The model under review builds one solid part; all positions refer to its coordinate system, in mm. Face numbers are marked on the shaded views. A direction names the side the tool comes from. Coordinates: 2 decimals unless noted, no trailing zeros. Order: outer loops, then holes, each group sorted by start corner. A loop starts at its lowest first (then second) coordinate and runs counter-clockwise, first axis right, second up. Notation, with made-up numbers: M 26,26 L 53,26 A12 cw 53,34 Z; hole C 73.25,21 d1. An arc over 180 degrees is marked long. One line per item, written item: value.
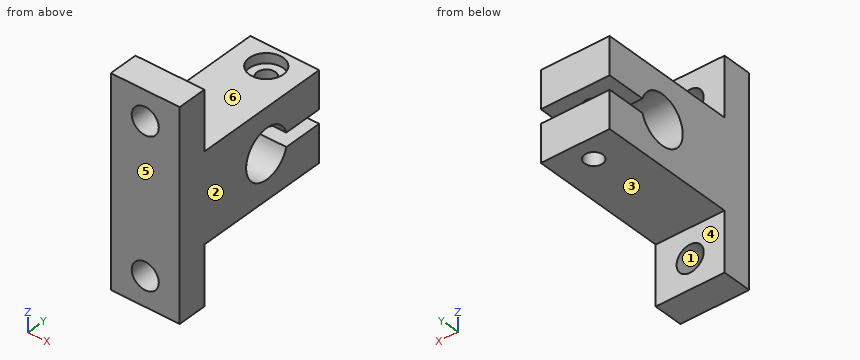
```python
from build123d import *

# Parameters (mm, degrees)
BOSS_EXTRUDE1_DEPTH = 14
SKETCH3_R           = 1.85
CUT_EXTRUDE1_DEPTH  = 48.455242071
SKETCH4_R           = 2.75
CUT_EXTRUDE2_DEPTH  = 53.383203415
SKETCH5_R           = 3.452522479
CUT_EXTRUDE3_DEPTH  = 2


with BuildPart() as part:
    # Sketch2 → Boss-Extrude1 (new body)
    with BuildSketch(Plane(origin=(0, 0, 0), x_dir=(0, 0, -1), z_dir=(1, 0, 0))):
        with BuildLine():
            Line((0, 0), (42, 0))
            Line((42, 0), (42, 6))
            Line((42, 6), (30, 6))
            Line((30, 6), (30, 34))
            Line((30, 34), (22.4, 34))
            Line((22.4, 34), (22.4, 26))
            ThreePointArc((22.4, 26), (21, 16.2), (19.6, 26))
            Line((19.6, 26), (19.6, 34))
            Line((19.6, 34), (12, 34))
            Line((12, 34), (12, 6))
            Line((12, 6), (0, 6))
            Line((0, 6), (0, 0))
        make_face()
    extrude(amount=BOSS_EXTRUDE1_DEPTH)

    # Sketch3 → Cut-Extrude1 (cut, through all)
    with BuildSketch(Plane(origin=(0, 0, -30), x_dir=(-1, 0, 0), z_dir=(0, 0, -1))):
        with Locations((-7, 29.5)):
            Circle(SKETCH3_R)
    extrude(amount=-CUT_EXTRUDE1_DEPTH, mode=Mode.SUBTRACT)

    # Sketch4 → Cut-Extrude2 (cut, through all)
    with BuildSketch(Plane(origin=(0, 6, 0), x_dir=(1, 0, 0), z_dir=(0, 1, 0))):
        with Locations(Location((7, 36, 0), (0, 0, 270))):
            Circle(SKETCH4_R)
        with Locations(Location((7, 6, 0), (0, 0, 270))):
            Circle(SKETCH4_R)
    extrude(amount=-CUT_EXTRUDE2_DEPTH, mode=Mode.SUBTRACT)

    # Sketch5 → Cut-Extrude3 (cut)
    with BuildSketch(Plane.XY.offset(-12)):
        with Locations((7, 29.5)):
            Circle(SKETCH5_R)
    extrude(amount=-CUT_EXTRUDE3_DEPTH, mode=Mode.SUBTRACT)


solid = part.part
```
(1) Tool access review of the marked faces 4, 5 and 6: name each direction out of +Z, -Z, +X, -X, +Y, -Y from which nothing blocks a thin tool from reaching the whole face with its end or side.
Geometry results:
face 4: -Z, +X, -X, +Y
face 5: +Z, -Z, +X, -X, -Y
face 6: +Z, +X, -X, +Y
(2) Insertion check: pin 1 Ø3.5 at (x, z) = (9.5, -35.5) entering from +Y; pin 2 Ø7 at (x, y) = (9.5, 14.5) entering from -Z; pin 3 Ø5.5 at (x, y) = (6, 30.5) entering from +Z. Each pin has a flat end and moves straight along its axis. Give the tip position at first contact, or say it passes through.
Geometry results:
pin 1: stops at y = 6
pin 2: stops at z = -30
pin 3: stops at z = -12
(3) We need section A-A, the plane x = 7. Count the separate pieces of the cut face and the enclosed holes in it, plus the area to 3 significant figures.
Geometry results:
separate pieces: 5
enclosed holes: 0
area: 527 mm2
(4) Mouldability with a two-part tool opening along X and no side actions: class the marked faces 1, 2 and 3 as +X half, -X half, draft (parallel to the pull), parting line (faces both ways), or undercut.
Geometry results:
face 1: undercut
face 2: +X half
face 3: draft
(5) We need section C-C, the plane y = 29.5. State the section outline as (x, z) points, plus the area to 3 significant figures.
Geometry results:
outline: M 0,-30 L 5.15,-30 L 5.15,-22.4 L 0,-22.4 Z; M 0,-19.6 L 5.15,-19.6 L 5.15,-14 L 3.55,-14 L 3.55,-12 L 0,-12 Z; M 8.85,-30 L 14,-30 L 14,-22.4 L 8.85,-22.4 Z; M 8.85,-19.6 L 14,-19.6 L 14,-12 L 10.45,-12 L 10.45,-14 L 8.85,-14 Z
area: 150 mm2
(6) For L1, parallel to Z at x = 5.75, y = 21.5; L2, parallel to Z at x = 9.5, y = 27; L3, parallel to Y at x = 8.25, z = -9, list the stretches that pass through material, from the lowest coordinate up.
Geometry results:
L1: z = -30 to -25.99, -16.01 to -12
L2: z = -30 to -22.4, -19.6 to -12
L3: y = 0 to 6
(7) We need section D-D, the plane y = 21.2. State the section outline as (x, z) points, plus the area to 3 significant figures.
Geometry results:
outline: M 0,-30 L 14,-30 L 14,-26 L 0,-26 Z; M 0,-16 L 14,-16 L 14,-12 L 0,-12 Z
area: 112 mm2
(8) We need section B-B, the plane z = -6. State the section outline as (x, y) points.
Geometry results:
outline: M 0,0 L 4.25,0 L 4.25,6 L 0,6 Z; M 9.75,0 L 14,0 L 14,6 L 9.75,6 Z
